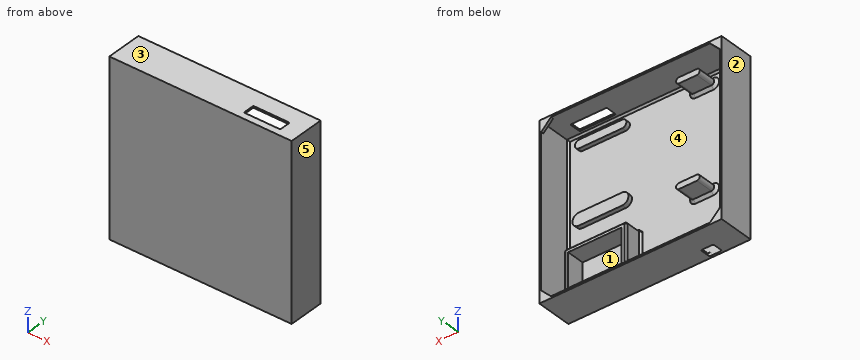
```python
from build123d import *

# Parameters (mm, degrees)
IZIM1_W                     = 204
IZIM1_H                     = 194
Y_KSEKLIK_EKSTR_ZYON2_DEPTH = 40
IZIM3_W                     = 200
IZIM3_H                     = 190
KES_EKSTR_ZYON2_DEPTH       = 37.5
Y_KSEKLIK_EKSTR_ZYON3_DEPTH = 23
IZIM6_W                     = 70
IZIM6_H                     = 48
IZIM6_W_2                   = 60
IZIM6_H_2                   = 38
Y_KSEKLIK_EKSTR_ZYON4_DEPTH = 20
Y_KSEKLIK_EKSTR_ZYON7_DEPTH = 5
Y_KSEKLIK_EKSTR_ZYON8_DEPTH = 3
KES_EKSTR_ZYON5_DEPTH       = 3
KES_EKSTR_ZYON7_DEPTH       = 3
PAH1_SIZE                   = 2
PAH2_SIZE                   = 3


with BuildPart() as part:
    # Çizim1 → Yükseklik-Ekstrüzyon2 (new body)
    with BuildSketch(Plane(origin=(0, 0, 0), x_dir=(1, 0, 0), z_dir=(0, 1, 0))):
        Rectangle(IZIM1_W, IZIM1_H)
    extrude(amount=Y_KSEKLIK_EKSTR_ZYON2_DEPTH)

    # Çizim3 → Kes-Ekstrüzyon2 (cut)
    with BuildSketch(Plane(origin=(0, 40, 0), x_dir=(1, 0, 0), z_dir=(0, 1, 0))):
        Rectangle(IZIM3_W, IZIM3_H)
    extrude(amount=-KES_EKSTR_ZYON2_DEPTH, mode=Mode.SUBTRACT)

    # Çizim4 → Yükseklik-Ekstrüzyon3 (add)
    with BuildSketch(Plane(origin=(0, 2.5, 0), x_dir=(1, 0, 0), z_dir=(0, 1, 0))):
        with BuildLine():
            Line((-62.5, 24.75), (-42.5, 24.75))
            ThreePointArc((-42.5, 24.75), (-39.25, 28), (-42.5, 31.25))
            Line((-42.5, 31.25), (-62.5, 31.25))
            ThreePointArc((-62.5, 31.25), (-65.75, 28), (-62.5, 24.75))
        make_face()
        with BuildLine():
            Line((-62.5, -87.25), (-42.5, -87.25))
            ThreePointArc((-42.5, -87.25), (-39.25, -84), (-42.5, -80.75))
            Line((-42.5, -80.75), (-62.5, -80.75))
            ThreePointArc((-62.5, -80.75), (-65.75, -84), (-62.5, -87.25))
        make_face()
    extrude(amount=Y_KSEKLIK_EKSTR_ZYON3_DEPTH)

    # Çizim6 → Yükseklik-Ekstrüzyon4 (add)
    with BuildSketch(Plane(origin=(0, 2.5, 0), x_dir=(1, 0, 0), z_dir=(0, 1, 0))):
        with Locations((54, 60)):
            Rectangle(IZIM6_W, IZIM6_H)
        with Locations((54, 60)):
            Rectangle(IZIM6_W_2, IZIM6_H_2, mode=Mode.SUBTRACT)
    extrude(amount=Y_KSEKLIK_EKSTR_ZYON4_DEPTH)

    # Çizim7 → Yükseklik-Ekstrüzyon7 (add)
    with BuildSketch(Plane(origin=(0, 2.5, 0), x_dir=(1, 0, 0), z_dir=(0, 1, 0))):
        with BuildLine():
            Line((35.6, -9.25), (84.4, -9.25))
            ThreePointArc((84.4, -9.25), (91.3, -2.35), (84.4, 4.55))
            Line((84.4, 4.55), (35.6, 4.55))
            ThreePointArc((35.6, 4.55), (28.7, -2.35), (35.6, -9.25))
        make_face()
        with BuildLine():
            Line((35.6, -77.25), (84.4, -77.25))
            ThreePointArc((84.4, -77.25), (88.64386759, -81.85), (84.4, -86.45))
            Line((84.4, -86.45), (35.6, -86.45))
            ThreePointArc((35.6, -86.45), (31, -81.85), (35.6, -77.25))
        make_face()
    extrude(amount=Y_KSEKLIK_EKSTR_ZYON7_DEPTH)

    # Çizim8 → Yükseklik-Ekstrüzyon8 (add)
    with BuildSketch(Plane(origin=(0, 40, 0), x_dir=(1, 0, 0), z_dir=(0, 1, 0))):
        Polygon((-102, 97), (-102, 82), (-87, 97), align=None)
        Polygon((102, 97), (87, 97), (102, 82), align=None)
        Polygon((102, -97), (102, -82), (87, -97), align=None)
        Polygon((-102, -97), (-87, -97), (-102, -82), align=None)
    extrude(amount=-Y_KSEKLIK_EKSTR_ZYON8_DEPTH)

    # Çizim9 → Kes-Ekstrüzyon5 (cut)
    with BuildSketch(Plane.XY.offset(97)):
        with BuildLine():
            Line((43.7, 7.5), (82, 7.5))
            ThreePointArc((82, 7.5), (82.848528137, 7.851471863), (83.2, 8.7))
            Line((83.2, 8.7), (83.2, 19.3))
            ThreePointArc((83.2, 19.3), (82.848528137, 20.148528137), (82, 20.5))
            Line((82, 20.5), (43.7, 20.5))
            ThreePointArc((43.7, 20.5), (42.851471863, 20.148528137), (42.5, 19.3))
            Line((42.5, 19.3), (42.5, 8.7))
            ThreePointArc((42.5, 8.7), (42.851471863, 7.851471863), (43.7, 7.5))
        make_face()
    extrude(amount=-KES_EKSTR_ZYON5_DEPTH, mode=Mode.SUBTRACT)

    # Çizim11 → Kes-Ekstrüzyon7 (cut)
    with BuildSketch(Plane(origin=(0, 0, -97), x_dir=(-1, 0, 0), z_dir=(0, 0, -1))):
        with BuildLine():
            Line((59.5, 2.5), (70.5, 2.5))
            ThreePointArc((70.5, 2.5), (71.560660172, 2.939339828), (72, 4))
            Line((72, 4), (72, 13))
            ThreePointArc((72, 13), (71.560660172, 14.060660172), (70.5, 14.5))
            Line((70.5, 14.5), (59.5, 14.5))
            ThreePointArc((59.5, 14.5), (58.439339828, 14.060660172), (58, 13))
            Line((58, 13), (58, 4))
            ThreePointArc((58, 4), (58.439339828, 2.939339828), (59.5, 2.5))
        make_face()
    extrude(amount=-KES_EKSTR_ZYON7_DEPTH, mode=Mode.SUBTRACT)

    # Pah1
    pah1_edges = [part.edges().sort_by_distance(p)[0] for p in [
        (0, 2.5, 95),
        (-100, 2.5, 0),
        (-85.25, 2.5, -95),
        (100, 2.5, 0),
        (20.25, 2.5, -95),
        (89, 22.5, -60),
        (54, 22.5, -84),
        (19, 22.5, -60),
        (54, 22.5, -36),
        (89, 2.5, -60),
        (89, 12.5, -36),
        (54, 2.5, -84),
        (89, 12.5, -84),
        (19, 2.5, -60),
        (19, 12.5, -84),
        (54, 2.5, -36),
        (19, 12.5, -36),
    ]]
    chamfer(pah1_edges, length=PAH1_SIZE)

    # Pah2
    pah2_edges = [part.edges().sort_by_distance(p)[0] for p in [
        (-39.25, 2.5, 84),
        (-52.5, 2.5, 80.75),
        (-65.75, 2.5, 84),
        (-52.5, 2.5, 87.25),
        (-65.75, 2.5, -28),
        (-52.5, 2.5, -24.75),
        (-39.25, 2.5, -28),
        (-52.5, 2.5, -31.25),
    ]]
    chamfer(pah2_edges, length=PAH2_SIZE)


solid = part.part
```
CAD build for the part. Positions are in the model's coordinates, mm. Face numbers are marked on the shaded views. A direction names the side the tool comes from. Round coordinates to 2 decimals unless told otherwise and drop trailing zeros. Order: outer loops, then holes, each group sorted by start corner. A loop starts at its lowest first (then second) coordinate and runs counter-clockwise, first axis right, second up. Notation, with made-up numbers: (-40, 68.25) - (-11, 68.25) arc R26 cw to (-11, 86.25) - close; hole circle Ø11 at (-32, 71). An arc over 180 degrees is marked (long way). Answer in a Markdown table with one row per item. Add a question column.
(1) 3-axis set-ups, long thin cutter, end or side, ignore diameter. For the marked faces 1 and 2: which of +Z, -Z, +X, -X, +Y, -Y reach the whole face in a straight line?
(2) Band-saw the part on D-D on z = -28. List the corners of the cut face in (x, y), and give its area (3 significant figures).
(3) Band-saw the part on C-C on x = -50.5. List the corners of the cut face in (y, z).
(4) Drop a flat-ended pin along its axis: pin 1 Ø4 at (x, z) = (72, -29) entering from +Y. Give the stop position or say it passes through.
(5) Probe L1, parallel to X at y = 6, z = -43; L2, parallel to Z at x = 22, y = 14; L3, parallel to Z at x = 55, y = 19.5. List the from-to ranges inside material, lowest first. Write a range as [from, to].
(6) Band-saw the part on B-B on z = 2.35. List the corners of the cut face in (x, y).
(7) Mould opens along X. For the marked faces 3, 4 and 5 say: +X half, -X half, draft (parallel to the pull), parting line (faces both ways), or undercut.
Data:
| question | item | result |
|---|---|---|
| 1 | face 1 | +Y |
| 1 | face 2 | +Z, -Z, -X, +Y, -Y |
| 2 | outline | (-102, 0) - (102, 0) - (102, 40) - (100, 40) - (100, 4.5) - (98, 2.5) - (-36.25, 2.5) - (-39.25, 5.5) - (-39.25, 25.5) - (-65.75, 25.5) - (-65.75, 5.5) - (-68.75, 2.5) - (-98, 2.5) - (-100, 4.5) - (-100, 40) - (-102, 40) - close |
| 2 | area | 1,280 mm^2 |
| 3 | outline | (0, -97) - (40, -97) - (40, -95) - (4.5, -95) - (2.5, -93) - (2.5, -34.25) - (5.5, -31.25) - (25.5, -31.25) - (25.5, -24.75) - (5.5, -24.75) - (2.5, -21.75) - (2.5, 77.75) - (5.5, 80.75) - (25.5, 80.75) - (25.5, 87.25) - (5.5, 87.25) - (2.5, 90.25) - (2.5, 93) - (4.5, 95) - (40, 95) - (40, 97) - (0, 97) - close |
| 4 | pin 1 | stops at y = 2.5 |
| 5 | L1 | x = [-102, -100], [19, 24], [84, 89], [100, 102] |
| 5 | L2 | z = [-97, -95], [-84, -36], [95, 97] |
| 5 | L3 | z = [-97, -95], [-84, -79], [-41, -36] |
| 6 | outline | (-102, 0) - (102, 0) - (102, 40) - (100, 40) - (100, 4.5) - (98, 2.5) - (91.3, 2.5) - (91.3, 7.5) - (28.7, 7.5) - (28.7, 2.5) - (-98, 2.5) - (-100, 4.5) - (-100, 40) - (-102, 40) - close |
| 7 | face 3 | draft |
| 7 | face 4 | undercut |
| 7 | face 5 | +X half |
